```python
from build123d import *

# Parameters (mm, degrees)
SKETCH_1_R          = 30
EXTRUDE_1_DEPTH     = 250
CUT_EXTRUDE_1_DEPTH = 254.574446662


with BuildPart() as part:
    # 草图1 → 凸台-拉伸1 (new body)
    with BuildSketch(Plane(origin=(0, 0, 0), x_dir=(1, 0, 0), z_dir=(0, 1, 0))):
        with Locations(Location((0, 0, 0), (0, 0, 270))):
            Circle(SKETCH_1_R)
    extrude(amount=EXTRUDE_1_DEPTH)

    # 草图3 → 切除-拉伸1 (cut, through all)
    with BuildSketch(Plane(origin=(0, 250, 0), x_dir=(1, 0, 0), z_dir=(0, 1, 0))):
        Polygon((25.531400595, -4.811193579), (16.93231616, 19.70524472), (-8.599084435, 24.516438299), (-25.531400595, 4.811193579), (-16.93231616, -19.70524472), (8.599084435, -24.516438299), align=None)
    extrude(amount=-CUT_EXTRUDE_1_DEPTH, mode=Mode.SUBTRACT)


solid = part.part
```
Part model, mm, in its own coordinate system. A direction names the side the tool comes from. Give positions to 0.01 mm unless a question says otherwise; leave off trailing zeros. Order: outer loops, then holes, each group sorted by start corner. A loop starts at its lowest first (then second) coordinate and runs counter-clockwise, first axis right, second up. Notation, with made-up numbers: M -16.75,35.25 L -2.75,35.25 A25 cw -2.75,57.25 Z; hole C -8,2.5 d11. An arc over 180 degrees is marked long. Use a Markdown table: item, result. Add a question column.
(1) Probe line 1 along Z through (x, y) = (-8.5, 178.5); line 2 along X through (y, z) = (177.5, 6); line 3 along X through (y, z) = (179, -4). List the from-to ranges inside material, lowest first. Write a range as [from, to].
(2) 3-axis set-ups, long thin cutter, end or side, ignore diameter. For faces 1 (the face through (4.6, 250, -22.4)), 2 (the face through (16.95, 126.75, 14.8)): which of +Z, -Z, +X, -X, +Y, -Y reach the whole face in a straight line?
(3) Saw through at C-C, the plane y = 76.5. Give the cut face in (x, z), and give its area (3 significant figures).
(4) Saw through at B-B, the plane z = 7.5. Give the cut face in (x, y).
(5) Drop flat-ended pins along their axis: P1, Ø2, axis at y = 28.5, z = -4.5, coming from the -X side; P2, Ø4, axis at y = 193.5, z = 22.5, coming from the +X side; P3, Ø12, axis at y = 53, z = -23, coming from the +X side. Give the stop position or say it passes through.
(6) Saw through at A-A, the plane x = 0. Give the cut face in (y, z), and give its area (3 significant figures).
(7) Mould opens along X. For faces 3 (the face through (4.6, 0, -22.4)), 4 (the face through (1.32, 123.25, -29.97)), 5 (the face through (21.29, 126.75, -7.28)) say: +X half, -X half, draft (parallel to the pull), parting line (faces both ways), or undercut.
Answer key:
| question | item | result |
|---|---|---|
| 1 | line 1 | [-28.77, -24.5], [21.29, 28.77] |
| 1 | line 2 | [-29.39, -21.74], [24.51, 29.39] |
| 1 | line 3 | [-29.73, -25.25], [22.44, 29.73] |
| 2 | face 1 | +Z, -Z, +X, -X, +Y |
| 2 | face 2 | +Y, -Y |
| 3 | outline | C 0,0 d60; hole M -25.53,-4.81 L -8.6,-24.52 L 16.93,-19.71 L 25.53,4.81 L 8.6,24.52 L -16.93,19.71 Z |
| 3 | area | 1,070 mm^2 |
| 4 | outline | M -29.05,0 L -21.21,0 L -21.21,250 L -29.05,250 Z; M 23.22,0 L 29.05,0 L 29.05,250 L 23.22,250 Z |
| 5 | P1 | x = -29.8 |
| 5 | P2 | x = 21.9 |
| 5 | P3 | x = 24.72 |
| 6 | outline | M 0,-30 L 250,-30 L 250,-22.9 L 0,-22.9 Z; M 0,22.9 L 250,22.9 L 250,30 L 0,30 Z |
| 6 | area | 3,550 mm^2 |
| 7 | face 3 | draft |
| 7 | face 4 | parting line |
| 7 | face 5 | undercut |
